The model under review builds one solid part; all positions refer to its coordinate system, in mm. Face numbers are marked on the shaded views. A direction names the side the tool comes from. Coordinates: 2 decimals unless noted, no trailing zeros. Order: outer loops, then holes, each group sorted by start corner. A loop starts at its lowest first (then second) coordinate and runs counter-clockwise, first axis right, second up. Notation, with made-up numbers: M -25,13 L 9,13 A20 ccw 9,51 Z; hole C -32,-2.75 d11. An arc over 180 degrees is marked long. Write each question's results on one line, items separated by ' | '.
from build123d import *

# Parameters (mm, degrees)
BOSS_EXTRUDE1_DEPTH = 50.8
SKETCH2_W           = 38.1
SKETCH2_H           = 38.1
CUT_EXTRUDE1_DEPTH  = 95.25
SKETCH3_W           = 76.2
SKETCH3_H           = 76.2
SKETCH3_W_2         = 50.8
SKETCH3_H_2         = 50.8
BOSS_EXTRUDE2_DEPTH = 6.35
FILLET1_R           = 2.54


with BuildPart() as part:
    # Sketch1 → Boss-Extrude1 (new body)
    with BuildSketch(Plane.XY):
        with BuildLine():
            Line((32.385, 107.95), (50.8, 107.95))
            Line((50.8, 107.95), (50.8, 0))
            Line((50.8, 0), (0, 0))
            Line((0, 0), (0, 107.95))
            Line((0, 107.95), (18.415, 107.95))
            ThreePointArc((18.415, 107.95), (25.4, 100.965), (32.385, 107.95))
        make_face()
    extrude(amount=BOSS_EXTRUDE1_DEPTH)

    # Sketch2 → Cut-Extrude1 (cut)
    with BuildSketch(Plane.XZ):
        with Locations((25.4, 25.4)):
            Rectangle(SKETCH2_W, SKETCH2_H)
    extrude(amount=-CUT_EXTRUDE1_DEPTH, mode=Mode.SUBTRACT)

    # Sketch3 → Boss-Extrude2 (add)
    with BuildSketch(Plane.XZ):
        with Locations((25.4, 25.4)):
            Rectangle(SKETCH3_W, SKETCH3_H)
        with Locations((25.4, 25.4)):
            Rectangle(SKETCH3_W_2, SKETCH3_H_2, mode=Mode.SUBTRACT)
    extrude(amount=-BOSS_EXTRUDE2_DEPTH)

    # Fillet1
    fillet1_edges = [part.edges().sort_by_distance(p)[0] for p in [
        (50.8, 6.35, 25.4),
        (25.4, 6.35, 50.8),
        (0, 6.35, 25.4),
        (25.4, 6.35, 0),
    ]]
    fillet(fillet1_edges, radius=FILLET1_R)


solid = part.part
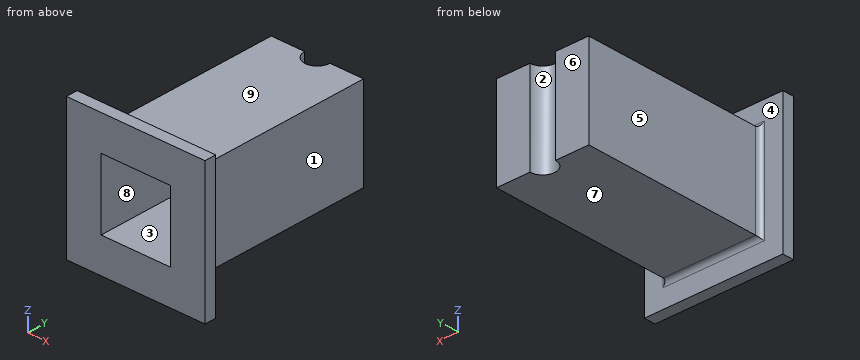
1) The part is to be moulded in two halves that separate along Z. For the marked faces 6, 7, 8 and 9, say which applies: pulls with the +Z half, pulls with the -Z half, needs draft (parallel to the pull), parting line crosses it, or undercut.
Solutions:
face 6: needs draft | face 7: pulls with the -Z half | face 8: undercut | face 9: pulls with the +Z half
2) For the marked faces 1, 2, 3, 4 and 5, list the 3-axis set-ups (+Z, -Z, +X, -X, +Y, -Y) from which the entire face can be reached by the end or side of a thin tool; tool diameter is ignored.
Solutions:
face 1: +Z, -Z, +X, +Y | face 2: +Z, -Z, +Y | face 3: -Y | face 4: +Y | face 5: +Z, -Z, -X, +Y
3) To check wall thickness, follow line 1 along X through (y, z) = (6, 25.5); line 2 along Z through (x, y) = (32.5, 51.5). State the ranges of each line that lie inside material, in increasing order.
Solutions:
line 1: -12.7 to 6.35, 44.45 to 63.5 | line 2: 0 to 6.35, 44.45 to 50.8
4) Take a section at C-C on z = 36. State the section outline as (x, y) points (3 decimals), plus the area to 3 significant figures.
Solutions:
outline: M -12.7,0 L 6.35,0 L 6.35,95.25 L 44.45,95.25 L 44.45,0 L 63.5,0 L 63.5,6.35 L 53.34,6.35 A2.54 cw 50.8,8.89 L 50.8,107.95 L 32.385,107.95 A6.985 cw 18.415,107.95 L 0,107.95 L 0,8.89 A2.54 cw -2.54,6.35 L -12.7,6.35 Z | area: 1,940 mm2
5) Take a section at A-A on x = 43. State the section outline as (y, z) points, plus the area to 3 significant figures.
Solutions:
outline: M 0,-12.7 L 6.35,-12.7 L 6.35,-2.54 A2.54 cw 8.89,0 L 107.95,0 L 107.95,50.8 L 8.89,50.8 A2.54 cw 6.35,53.34 L 6.35,63.5 L 0,63.5 L 0,44.45 L 95.25,44.45 L 95.25,6.35 L 0,6.35 Z | area: 2,020 mm2
6) Take a section at D-D on z = 5. State the section outline as (x, y) points (3 decimals), plus the area to 3 significant figures.
Solutions:
outline: M -12.7,0 L 63.5,0 L 63.5,6.35 L 53.34,6.35 A2.54 cw 50.8,8.89 L 50.8,107.95 L 32.385,107.95 A6.985 cw 18.415,107.95 L 0,107.95 L 0,8.89 A2.54 cw -2.54,6.35 L -12.7,6.35 Z | area: 5,570 mm2
7) For pin 1 (19 mm diameter, centred on x = 24, y = 35, fed in from -Z); pin 2 (1 mm diameter, centred on x = 27, z = 34, fed in from +Y); pin 3 (12 mm diameter, centred on x = -0.5, y = 47.5, fed in from +Z); pin 4 (1 mm diameter, centred on x = 39, z = 2.5, fed in from -Y), all flat-tipped, find the tip position at first contact; note any pin that passes through.
Solutions:
pin 1: z = 0 | pin 2: y = 101.29 | pin 3: z = 50.8 | pin 4: y = 0
8) Take a section at B-B on y = 37.5. State the section outline as (x, z) points.
Solutions:
outline: M 0,0 L 50.8,0 L 50.8,50.8 L 0,50.8 Z; hole M 6.35,6.35 L 44.45,6.35 L 44.45,44.45 L 6.35,44.45 Z
